from build123d import *
from build123d.topology import SkipClean

# Parameters (mm, degrees)
SKETCH1_W            = 39
SKETCH1_H            = 23.712741858
BOSS_EXTRUDE1_DEPTH  = 2
SKETCH9_R            = 4.05
CUT_EXTRUDE6_DEPTH   = 5
SKETCH10_R           = 1.25
BOSS_EXTRUDE5_DEPTH  = 5.5
SKETCH11_R           = 2.5
CUT_EXTRUDE7_DEPTH   = 5
BOSS_EXTRUDE6_START  = -5.5
SKETCH12_R           = 2.5
BOSS_EXTRUDE6_DEPTH  = 5.5
BOSS_EXTRUDE7_DEPTH  = 28
BOSS_EXTRUDE8_START  = 2
SKETCH14_W           = 39
SKETCH14_H           = 29
SKETCH14_R           = 1.25
SKETCH14_R_2         = 4.05
BOSS_EXTRUDE8_DEPTH  = 2
SKETCH15_R           = 3
CUT_EXTRUDE8_DEPTH   = 2
BOSS_EXTRUDE9_DEPTH  = 5
BOSS_EXTRUDE10_START = 5
BOSS_EXTRUDE10_DEPTH = 5
CUT_EXTRUDE9_REACH   = 41.579
SKETCH18_W           = 39
SKETCH18_H           = 30
SKETCH19_W           = 10.5
SKETCH19_H           = 39
BOSS_EXTRUDE11_DEPTH = 5
SKETCH20_W           = 10.5
SKETCH20_H           = 39
BOSS_EXTRUDE12_DEPTH = 5


with BuildPart() as part:
    # Sketch1 → Boss-Extrude1 (new body)
    with BuildSketch(Plane.XY):
        with Locations((0, -11)):
            Rectangle(SKETCH1_W, SKETCH1_H)
        with BuildLine():
            ThreePointArc((1.25, -19), (0, -17.75), (-1.25, -19))
            ThreePointArc((-1.25, -19), (0, -20.25), (1.25, -19))
        make_face(mode=Mode.SUBTRACT)
        with BuildLine():
            ThreePointArc((-6.75, -11), (-8, -9.75), (-9.25, -11))
            ThreePointArc((-9.25, -11), (-8, -12.25), (-6.75, -11))
        make_face(mode=Mode.SUBTRACT)
        with BuildLine():
            ThreePointArc((1.25, -3), (0, -1.75), (-1.25, -3))
            ThreePointArc((-1.25, -3), (0, -4.25), (1.25, -3))
        make_face(mode=Mode.SUBTRACT)
        with BuildLine():
            ThreePointArc((9.25, -11), (8, -9.75), (6.75, -11))
            ThreePointArc((6.75, -11), (8, -12.25), (9.25, -11))
        make_face(mode=Mode.SUBTRACT)
    extrude(amount=BOSS_EXTRUDE1_DEPTH)

    # Sketch9 → Cut-Extrude6 (cut)
    with BuildSketch(Plane.XY.offset(2)):
        with Locations((0, -11)):
            Circle(SKETCH9_R)
    extrude(amount=-CUT_EXTRUDE6_DEPTH, mode=Mode.SUBTRACT)

    # Sketch10 → Boss-Extrude5 (add)
    # profile 1 of 2: a face of its own
    with BuildSketch(Plane.ZY.offset(19.5)):
        with BuildLine():
            Line((4.2, 3.5), (8.5, 3.5))
            Line((8.5, 3.5), (8.5, 0.5))
            ThreePointArc((8.5, 0.5), (7.474873734, -1.974873734), (5, -3))
            Line((5, -3), (2, -3))
            Line((2, -3), (2, 0.856370929))
            Line((2, 0.856370929), (0, 0.856370929))
            Line((0, 0.856370929), (0, 3.5))
            Line((0, 3.5), (4.2, 3.5))
        make_face()
        with Locations((5.25, 0.25)):
            Circle(SKETCH10_R, mode=Mode.SUBTRACT)
    # profile 2 of 2: a face of its own
    with BuildSketch(Plane.ZY.offset(19.5)):
        with BuildLine():
            Line((5, -19), (2, -19))
            Line((2, -19), (2, -22.856370929))
            Line((2, -22.856370929), (0, -22.856370929))
            Line((0, -22.856370929), (0, -25.5))
            Line((0, -25.5), (4.2, -25.5))
            Line((4.2, -25.5), (8.5, -25.5))
            Line((8.5, -25.5), (8.5, -22.5))
            ThreePointArc((8.5, -22.5), (7.474873734, -20.025126266), (5, -19))
        make_face()
        with Locations((5.25, -22.25)):
            Circle(SKETCH10_R, mode=Mode.SUBTRACT)
    extrude(amount=-BOSS_EXTRUDE5_DEPTH)

    # Sketch11 → Cut-Extrude7 (cut)
    with BuildSketch(Plane.ZY.offset(19.5)):
        with Locations((5.25, 0.25)):
            Circle(SKETCH11_R)
        with Locations(Location((5.25, -22.25, 0), (0, 0, 180))):
            Circle(SKETCH11_R)
    extrude(amount=-CUT_EXTRUDE7_DEPTH, mode=Mode.SUBTRACT)

    # Sketch12 → Boss-Extrude6 (add)
    with BuildSketch(Plane(origin=(19.5, 0, 0), x_dir=(0, 0, -1), z_dir=(1, 0, 0)).offset(BOSS_EXTRUDE6_START)):
        with BuildLine():
            ThreePointArc((-8.5, 0.5), (-7.474873734, -1.974873734), (-5, -3))
            Line((-5, -3), (-2, -3))
            Line((-2, -3), (-2, -19))
            Line((-2, -19), (-5, -19))
            ThreePointArc((-5, -19), (-7.474873734, -20.025126266), (-8.5, -22.5))
            Line((-8.5, -22.5), (-8.5, -25.5))
            Line((-8.5, -25.5), (0, -25.5))
            Line((0, -25.5), (0, 3.5))
            Line((0, 3.5), (-8.5, 3.5))
            Line((-8.5, 3.5), (-8.5, 0.5))
        make_face()
        with Locations((-5.25, -22.25)):
            Circle(SKETCH12_R, mode=Mode.SUBTRACT)
        with Locations(Location((-5.25, 0.25, 0), (0, 0, 180))):
            Circle(SKETCH12_R, mode=Mode.SUBTRACT)
    extrude(amount=BOSS_EXTRUDE6_DEPTH)

    # Sketch13 → Boss-Extrude7 (add)
    with BuildSketch(Plane.ZY.offset(-14)):
        Polygon((0, 3.5), (4.2, 3.5), (2, 1.3), (2, 0.856370929), (0, 0.856370929), align=None)
        Polygon((2, -22.856370929), (0, -22.856370929), (0, -25.5), (4.2, -25.5), (2, -23.3), align=None)
    extrude(amount=BOSS_EXTRUDE7_DEPTH)

    # Sketch14 → Boss-Extrude8 (add)
    with SkipClean():  # the faces are left unmerged after this step: merging them gives an invalid solid
        with BuildSketch(Plane(origin=(0, 0, 0), x_dir=(-1, 0, 0), z_dir=(0, 0, -1)).offset(BOSS_EXTRUDE8_START)):
            with Locations((0, -11)):
                Rectangle(SKETCH14_W, SKETCH14_H)
            with Locations((0, -19)):
                Circle(SKETCH14_R, mode=Mode.SUBTRACT)
            with Locations((8, -11)):
                Circle(SKETCH14_R, mode=Mode.SUBTRACT)
            with Locations((0, -3)):
                Circle(SKETCH14_R, mode=Mode.SUBTRACT)
            with Locations(Location((0, -11, 0), (0, 0, 180))):
                Circle(SKETCH14_R_2, mode=Mode.SUBTRACT)
            with Locations((-8, -11)):
                Circle(SKETCH14_R, mode=Mode.SUBTRACT)
        extrude(amount=-BOSS_EXTRUDE8_DEPTH)

    # Sketch15 → Cut-Extrude8 (cut)
    with BuildSketch(Plane.XY.offset(2)):
        with Locations((0, -3)):
            Circle(SKETCH15_R)
        with Locations((8, -11)):
            Circle(SKETCH15_R)
        with Locations((0, -19)):
            Circle(SKETCH15_R)
        with Locations((-8, -11)):
            Circle(SKETCH15_R)
    extrude(amount=-CUT_EXTRUDE8_DEPTH, mode=Mode.SUBTRACT)

    # Sketch16 → Boss-Extrude9 (add)
    with BuildSketch(Plane(origin=(0, 3.5, 0), x_dir=(1, 0, 0), z_dir=(0, 1, 0))):
        with BuildLine():
            ThreePointArc((-19.5, -8.5), (-17.889087297, -12.389087297), (-14, -14))
            Line((-14, -14), (14, -14))
            ThreePointArc((14, -14), (17.889087297, -12.389087297), (19.5, -8.5))
            Line((19.5, -8.5), (14, -8.5))
            Line((14, -8.5), (14, -4.2))
            Line((14, -4.2), (-14, -4.2))
            Line((-14, -4.2), (-14, -8.5))
            Line((-14, -8.5), (-19.5, -8.5))
        make_face()
        Polygon((-19.5, -8.5), (-14, -8.5), (-14, -4.2), (14, -4.2), (14, -8.5), (19.5, -8.5), (19.5, 2), (-19.5, 2), align=None)
    extrude(amount=BOSS_EXTRUDE9_DEPTH)

    # Sketch17 → Boss-Extrude10 (add)
    with BuildSketch(Plane.XZ.offset(25.5).offset(BOSS_EXTRUDE10_START)):
        with BuildLine():
            Line((19.5, -2), (19.5, 8.5))
            ThreePointArc((19.5, 8.5), (17.889087297, 12.389087297), (14, 14))
            Line((14, 14), (-14, 14))
            ThreePointArc((-14, 14), (-17.889087297, 12.389087297), (-19.5, 8.5))
            Line((-19.5, 8.5), (-19.5, -2))
            Line((-19.5, -2), (19.5, -2))
        make_face()
    extrude(amount=-BOSS_EXTRUDE10_DEPTH)

    # Cut-Extrude9: up to this face of the body (flat: up to its plane)
    cut_extrude9_end = Plane(part.part.faces().sort_by_distance((16.75, -3.461103025, 2))[0])
    # Sketch18 → Cut-Extrude9 (cut, up to the picked face)
    with BuildSketch(Plane.XY.offset(14), mode=Mode.PRIVATE) as cut_extrude9_sk1:
        with Locations((0, -11)):
            Rectangle(SKETCH18_W, SKETCH18_H)
    cut_extrude9_tool1 = split(extrude(cut_extrude9_sk1.sketch, amount=-CUT_EXTRUDE9_REACH, mode=Mode.PRIVATE), bisect_by=cut_extrude9_end, keep=Keep.BOTH, mode=Mode.PRIVATE)
    add(cut_extrude9_tool1.solids().sort_by(Axis((0, -11, 14), (0, 0, -1)))[0], mode=Mode.SUBTRACT)

    # Sketch19 → Boss-Extrude11 (add)
    with BuildSketch(Plane.ZY.offset(19.5)):
        with Locations((3.25, -11)):
            Rectangle(SKETCH19_W, SKETCH19_H)
    extrude(amount=BOSS_EXTRUDE11_DEPTH)

    # Sketch20 → Boss-Extrude12 (add)
    with BuildSketch(Plane(origin=(19.5, 0, 0), x_dir=(0, 0, -1), z_dir=(1, 0, 0))):
        with Locations((-3.25, -11)):
            Rectangle(SKETCH20_W, SKETCH20_H)
    extrude(amount=BOSS_EXTRUDE12_DEPTH)


solid = part.part
Verification items for the finished model (mm, model axes). A direction names the side the tool comes from. Round coordinates to 2 decimals unless told otherwise and drop trailing zeros. Loops run counter-clockwise (first coordinate to the right, second up) from the corner with the lowest first, then second, coordinate; pieces in that order, holes last. Notation, with made-up numbers: (-13, -27.5) - (3, -27.5) arc R22 cw to (3, 6.5) - close; hole circle Ø10 at (76, -12). An arc over 180 degrees is marked (long way). Answer in a Markdown table with one row per item. Add a question column.
Q1. Release check for a two-part mould opening along Y. For faces 1 (the face through (0, 8.5, 6)), 2 (the face through (22, -11, 8.5)), 3 (the face through (19.5, -11, 5)), 4 (the face through (0, -30.5, 6)) record: pulls with the +Y half, pulls with the -Y half, needs draft (parallel to the pull), parting line crosses it, or undercut.
Q2. Gauge pin test, flat ends, axial feed: pin 1 (1.5 mm diameter, centred on x = 0, y = -3, fed in from -Z); pin 2 (4 mm diameter, centred on x = 8, y = -11, fed in from +Z); pin 3 (3 mm diameter, centred on x = -14.5, y = 2, fed in from +Z); pin 4 (5.5 mm diameter, centred on x = -21.5, y = -3.5, fed in from +Z). Record the tip position at first contact, or that the pin passes through.
Q3. Material ranges on line 1 (Y direction, x = 0, z = -0.85); line 2 (X direction, y = -11, z = -1.1); line 3 (Y direction, x = 0, z = 0.95), recorded low to high.
Q4. Section check B-B on y = -3. Enter the section's corners in (x, z).
Q5. Section check A-A on x = 8. Enter the section's corners in (y, z).
Q6. Section check D-D on z = 6.25. Enter the section's corners in (x, y).
Q7. Tool access check on faces 5 (the face through (0, -26, 8)), 6 (the face through (17.93, -28.28, 12.35)). Record the directions out of +Z, -Z, +X, -X, +Y, -Y that give a thin tool (end or side, any length) a straight path to the whole face; none if there is none.
Q8. Section check C-C on y = -11. Enter the section's corners in (x, z).
Found:
| question | item | result |
|---|---|---|
| 1 | face 1 | pulls with the +Y half |
| 1 | face 2 | needs draft |
| 1 | face 3 | undercut |
| 1 | face 4 | pulls with the -Y half |
| 2 | pin 1 | passes through |
| 2 | pin 2 | stops at z = 0 |
| 2 | pin 3 | stops at z = 2 |
| 2 | pin 4 | stops at z = 8.5 |
| 3 | line 1 | y = -30.5 to -20.25, -17.75 to -15.05, -6.95 to -4.25, -1.75 to 8.5 |
| 3 | line 2 | x = -24.5 to -9.25, -6.75 to -4.05, 4.05 to 6.75, 9.25 to 24.5 |
| 3 | line 3 | y = -30.5 to -22, -16 to -15.05, -6.95 to -6, 0 to 8.5 |
| 4 | outline | (-24.5, -2) - (-1.25, -2) - (-1.25, 0) - (-3, 0) - (-3, 2) - (-19.5, 2) - (-19.5, 8.5) - (-24.5, 8.5) - close; (1.25, -2) - (24.5, -2) - (24.5, 8.5) - (19.5, 8.5) - (19.5, 2) - (3, 2) - (3, 0) - (1.25, 0) - close |
| 5 | outline | (-30.5, -2) - (-12.25, -2) - (-12.25, 0) - (-14, 0) - (-14, 2) - (-26, 2) - (-26, 14) - (-30.5, 14) - close; (-9.75, -2) - (8.5, -2) - (8.5, 14) - (4, 14) - (4, 2) - (-8, 2) - (-8, 0) - (-9.75, 0) - close |
| 6 | outline | (-24.5, -30.5) - (24.5, -30.5) - (24.5, 8.5) - (-24.5, 8.5) - close; hole (-19.5, -26) - (19.5, -26) - (19.5, 4) - (-19.5, 4) - close |
| 7 | face 5 | +Z |
| 7 | face 6 | +Z, +X, +Y, -Y |
| 8 | outline | (-24.5, -2) - (-9.25, -2) - (-9.25, 0) - (-11, 0) - (-11, 2) - (-19.5, 2) - (-19.5, 8.5) - (-24.5, 8.5) - close; (-6.75, -2) - (-4.05, -2) - (-4.05, 2) - (-5, 2) - (-5, 0) - (-6.75, 0) - close; (4.05, -2) - (6.75, -2) - (6.75, 0) - (5, 0) - (5, 2) - (4.05, 2) - close; (9.25, -2) - (24.5, -2) - (24.5, 8.5) - (19.5, 8.5) - (19.5, 2) - (11, 2) - (11, 0) - (9.25, 0) - close |
